Geometry: final body of the model. Coordinates: model frame, mm. Coordinates: 2 decimals unless noted, no trailing zeros. Write each loop counter-clockwise with the first axis right and the second up, starting at its lowest first coordinate (ties: lowest second). Pieces come first, ordered by that corner, then holes. Notation, with made-up numbers: (-12, 36) - (-5, 36) arc R29 ccw to (-5, 59) - close; hole circle Ø5 at (15, -8.75). An arc over 180 degrees is marked (long way). Answer as a JSON object with one key per item and string values. Group by question number.
Item 1: Section B-B on y = -27.5. Return loops of the section in (x, z).
Item 2: First-contact query: pin 1 Ø4.5 at (x, y) = (-47.5, -27.5) entering from +Z; pin 2 Ø2 at (x, y) = (-17.5, 26.5) entering from -Z; pin 3 Ø4 at (x, y) = (47.5, 27.5) entering from +Z. Flat tips, straight axial feed; report the tip coordinate or a pass-through.
Item 3: Section A-A on x = -17.5. Return loops of the section in (y, z), and give its area (3 significant figures).
Item 4: Line query: line 1 along Y through (x, z) = (40.5, 1.6); line 2 along Y through (x, z) = (47.5, 1.1); line 3 along X through (y, z) = (-27.5, 1.75). Output: solid intervals per line, ascending. Write a range as from..to.
Item 5: Section C-C on x = 47.5. Return loops of the section in (y, z), and give its area (3 significant figures).
Item 6: Mould query, pull axis X, two halves, no side actions, for faces 1 (the flat face through (-1, -32.5, 2)), 2 (the flat face through (-52.5, 0, 2)), 3 (the cylindrical face through (-18.655, -22.979, 1.972)). Classes: pulls with the +X half, pulls with the -X half, needs draft (parallel to the pull), parting line crosses it, or undercut.
```python
from build123d import *

# Parameters (mm, degrees)
SKETCH_1_W                     = 105
SKETCH_1_H                     = 65
EXTRUDE_1_DEPTH                = 4
HOLE_WIZARD_M3_1_D             = 2.5
HOLE_WIZARD_M3_1_2_D           = 3.4
HOLE_WIZARD_M3_1_2_CSINK_D     = 6.3
HOLE_WIZARD_M3_1_2_CSINK_ANGLE = 90


with BuildPart() as part:
    # 草圖1 → 填料-伸長1 (new body)
    with BuildSketch(Plane.XY):
        Rectangle(SKETCH_1_W, SKETCH_1_H)
    extrude(amount=EXTRUDE_1_DEPTH)

    # Hole Wizard M3 _1 (through all)
    with Locations(Plane.XY.offset(4)):
        with Locations((40.5, 26.5), (40.5, -22.5), (-17.5, -22.5), (-17.5, 26.5)):
            Hole(HOLE_WIZARD_M3_1_D / 2)

    # Hole Wizard M3 _1 2 (through all)
    with Locations(Plane.XY.offset(4)):
        with Locations((-47.5, 27.5), (-47.5, -27.5), (47.5, 27.5), (47.5, -27.5)):
            CounterSinkHole(HOLE_WIZARD_M3_1_2_D / 2, HOLE_WIZARD_M3_1_2_CSINK_D / 2, counter_sink_angle=HOLE_WIZARD_M3_1_2_CSINK_ANGLE)


solid = part.part
```
Checks:
{
 "1": {"outline": "(-52.5, 0) - (-49.2, 0) - (-49.2, 2.55) - (-50.65, 4) - (-52.5, 4) - close; (-45.8, 0) - (45.8, 0) - (45.8, 2.55) - (44.35, 4) - (-44.35, 4) - (-45.8, 2.55) - close; (49.2, 0) - (52.5, 0) - (52.5, 4) - (50.65, 4) - (49.2, 2.55) - close"},
 "2": {"pin 1": "z = 3.1", "pin 2": "through", "pin 3": "z = 2.85"},
 "3": {"outline": "(-32.5, 0) - (-23.75, 0) - (-23.75, 4) - (-32.5, 4) - close; (-21.25, 0) - (25.25, 0) - (25.25, 4) - (-21.25, 4) - close; (27.75, 0) - (32.5, 0) - (32.5, 4) - (27.75, 4) - close", "area": "240 mm^2"},
 "4": {"line 1": "-32.5..-23.75, -21.25..25.25, 27.75..32.5", "line 2": "-32.5..-29.2, -25.8..25.8, 29.2..32.5", "line 3": "-52.5..-49.2, -45.8..45.8, 49.2..52.5"},
 "5": {"outline": "(-32.5, 0) - (-29.2, 0) - (-29.2, 2.55) - (-30.65, 4) - (-32.5, 4) - close; (-25.8, 0) - (25.8, 0) - (25.8, 2.55) - (24.35, 4) - (-24.35, 4) - (-25.8, 2.55) - close; (29.2, 0) - (32.5, 0) - (32.5, 4) - (30.65, 4) - (29.2, 2.55) - close", "area": "229 mm^2"},
 "6": {"face 1": "needs draft", "face 2": "pulls with the -X half", "face 3": "undercut"}
}
